Autodesk Inventor part; units mm, degrees
ref_plane "YZ Plane" through (0, 0, 0) normal (1, 0, 0) x (0, 1, 0)
ref_plane "XZ Plane" through (0, 0, 0) normal (0, 1, 0) x (-1, 0, 0)
ref_plane "XY Plane" through (0, 0, 0) normal (0, 0, 1) x (1, 0, 0)
sketch "Sketch1" plane through (0, 0, 0) normal (0, 0, 1) x (1, 0, 0)
  line L0 (0, 0) -> (170, 0)
  line L1 (170, 0) -> (170, 170)
  line L2 (170, 170) -> (0, 170)
  line L3 (0, 170) -> (0, 0)
  dimension "d0" = 170
  dimension "d1" = 170
extrude "Extrusion1" add sketch "Sketch1" along normal blind 10
sketch "Sketch2" plane through (0, 0, 10) normal (0, 0, 1) x (1, 0, 0)
  line L0 (170, 170) -> (0, 170)
  line L1 (0, 170) -> (0, 155)
  line L2 (0, 170) -> (0, 0)
  line L3 (0, 0) -> (170, 0)
  line L4 (0, 0) -> (0, 15)
  line L5 (0, 15) -> (155, 15)
  line L6 (155, 15) -> (155, 155)
  line L7 (155, 155) -> (15, 155)
  line L8 (15, 155) -> (15, 15)
  line L9 (15, 155) -> (30, 155)
  circle A0 centre (15, 155) radius 7.5
  circle A1 centre (155, 155) radius 7.5
  circle A2 centre (155, 15) radius 7.5
  circle A3 centre (15, 15) radius 7.5
  dimension "d4" = 15
  dimension "d5" = 15
  dimension "d6" = 155
  dimension "d7" = 140
  dimension "d8" = 140
  dimension "d9" = 140
  dimension "d10" = 15
  dimension "d11" = 15
  dimension "d12" = 15
  dimension "d13" = 15
extrude "Extrusion2" cut sketch "Sketch2" against normal blind 10 contours L8 A3 L5 | L5 A3 | L5 A3 L8 | A2 L6 L5 | L5 L6 A2 | A0 L7 L8 | L8 L7 A0 | A1 L7 L6 | L6 L7 A1
sketch "Sketch3" plane through (0, 0, 10) normal (0, 0, 1) x (1, 0, 0)
  line L0 (170, 170) -> (0, 170)
  line L1 (0, 170) -> (85, 170)
  line L2 (85, 170) -> (85, 85)
  circle A0 centre (85, 85) radius 7.5
  point P0 (0, 0)
  dimension "d16" = 85
  dimension "d17" = 85
  dimension "d18" = 15
extrude "Extrusion3" cut sketch "Sketch3" against normal blind 10
properties part number "AB"
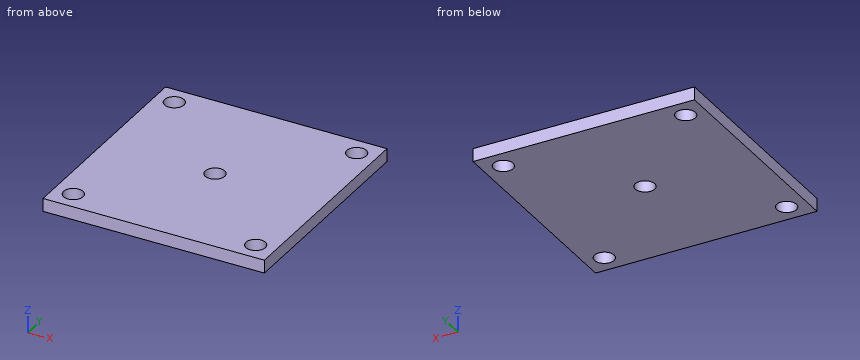
Design review of the part built by this model. Coordinates are the model's own, in mm. Coordinates: 2 decimals unless noted, no trailing zeros. Write each loop counter-clockwise with the first axis right and the second up, starting at its lowest first coordinate (ties: lowest second). Pieces come first, ordered by that corner, then holes. Notation, with made-up numbers: (24.25, 49.5) - (76.25, 49.5) arc R36 cw to (76.25, 88.5) - close; hole circle Ø8 at (-24, 68.25). An arc over 180 degrees is marked (long way). One line per item, written item: value.
1) Add section A-A (y = 85). State the section outline as (x, z) points.
Answer sheet:
outline: (0, 0) - (77.5, 0) - (77.5, 10) - (0, 10) - close; (92.5, 0) - (170, 0) - (170, 10) - (92.5, 10) - close
2) To check wall thickness, follow probe 1 along Y at (x, z) = (155, 5); probe 2 along Y at (x, z) = (19, 2.75). State the ranges of each line that lie inside material, in increasing order.
Answer sheet:
probe 1: y = 0 to 7.5, 22.5 to 147.5, 162.5 to 170
probe 2: y = 0 to 8.66, 21.34 to 148.66, 161.34 to 170
3) Add section D-D (z = 2.75). State the section outline as (x, y) points, plus the area to 3 significant figures.
Answer sheet:
outline: (0, 0) - (170, 0) - (170, 170) - (0, 170) - close; hole circle Ø15 at (15, 15); hole circle Ø15 at (15, 155); hole circle Ø15 at (85, 85); hole circle Ø15 at (155, 15); hole circle Ø15 at (155, 155)
area: 28,000 mm2
4) Add section B-B (x = 155). State the section outline as (y, z) points, plus the area to 3 significant figures.
Answer sheet:
outline: (0, 0) - (7.5, 0) - (7.5, 10) - (0, 10) - close; (22.5, 0) - (147.5, 0) - (147.5, 10) - (22.5, 10) - close; (162.5, 0) - (170, 0) - (170, 10) - (162.5, 10) - close
area: 1,400 mm2
